from build123d import *

# Parameters (mm, degrees)
SKETCH1_W           = 80
SKETCH1_H           = 24.7
BOSS_EXTRUDE1_DEPTH = 1
CUT_EXTRUDE1_DEPTH  = 100
CUT_EXTRUDE2_DEPTH  = 1
BOSS_EXTRUDE2_START = -80
BOSS_EXTRUDE2_DEPTH = 80


with BuildPart() as part:
    # Sketch1 → Boss-Extrude1 (new body)
    with BuildSketch(Plane.XY):
        Rectangle(SKETCH1_W, SKETCH1_H)
    extrude(amount=BOSS_EXTRUDE1_DEPTH)

    # Sketch2 → Cut-Extrude1 (cut)
    with BuildSketch(Plane.ZY.offset(40)):
        with BuildLine():
            Line((0, -12.35), (1, -12.35))
            ThreePointArc((1, -12.35), (0.292893219, -12.057106781), (0, -11.35))
            Line((0, -11.35), (0, -12.35))
        make_face()
    extrude(amount=-CUT_EXTRUDE1_DEPTH, mode=Mode.SUBTRACT)

    # Sketch3 → Cut-Extrude2 (cut)
    with BuildSketch(Plane(origin=(0, 0, 0), x_dir=(-1, 0, 0), z_dir=(0, 0, -1))):
        with BuildLine():
            Line((34, 7.35), (16, 7.35))
            ThreePointArc((16, 7.35), (15.292893219, 7.057106781), (15, 6.35))
            Line((15, 6.35), (15, -1.65))
            ThreePointArc((15, -1.65), (15.292893219, -2.357106781), (16, -2.65))
            Line((16, -2.65), (34, -2.65))
            ThreePointArc((34, -2.65), (34.707106781, -2.357106781), (35, -1.65))
            Line((35, -1.65), (35, 6.35))
            ThreePointArc((35, 6.35), (34.707106781, 7.057106781), (34, 7.35))
        make_face()
    extrude(amount=-CUT_EXTRUDE2_DEPTH, mode=Mode.SUBTRACT)

    # Sketch4 → Boss-Extrude2 (add)
    with BuildSketch(Plane(origin=(40, 0, 0), x_dir=(0, 0, -1), z_dir=(1, 0, 0)).offset(BOSS_EXTRUDE2_START)):
        with BuildLine():
            Line((-1, -12.49), (-1, -12.35))
            ThreePointArc((-1, -12.35), (-0.292893219, -12.057106781), (0, -11.35))
            Line((0, -11.35), (0.14, -11.35))
            ThreePointArc((0.14, -11.35), (-0.193898269, -12.156101731), (-1, -12.49))
        make_face()
    extrude(amount=BOSS_EXTRUDE2_DEPTH)


solid = part.part
Geometry: final body of the model. Coordinates: model frame, mm. A direction names the side the tool comes from. Give positions to 0.01 mm unless a question says otherwise; leave off trailing zeros. Write each loop counter-clockwise with the first axis right and the second up, starting at its lowest first coordinate (ties: lowest second). Pieces come first, ordered by that corner, then holes.
(1) Cut plane A-A, the plane y = 5.25. Return loops of the section in (x, z), then the cut area to 3 significant figures.
(2) Cut plane D-D, the plane x = -6.5. Return loops of the section in (y, z).
(3) Cut plane B-B, the plane x = -28. Return loops of the section in (y, z), then the cut area to 3 significant figures.
(4) Cut plane C-C, the plane z = 0.4. Return loops of the section in (x, y).
(5) Access query for faces 1 (the flat face through (-1, 0, 1)), 2 (the flat face through (-1, 1, 0)). Directions: +Z, -Z, +X, -X, +Y, -Y. A direction counts if a zero-diameter tool reaches every point of the face in a straight line with its end or side. Return the directions, or none.
(6) Ray query, line 1 (X direction, y = 3, z = 0.4); line 2 (Y direction, x = -3.5, z = 0.9); line 3 (Z direction, x = 23, y = -4.5). Return the intervals inside material, ascending.
Values follow:
1. outline: (-40, 0) - (-35, 0) - (-35, 1) - (-40, 1) - close; (-15, 0) - (40, 0) - (40, 1) - (-15, 1) - close
1. area: 60.0 mm2
2. outline: (-12.49, 1) arc R1.14 ccw to (-11.35, -0.14) - (-11.35, 0) - (12.35, 0) - (12.35, 1) - close
3. outline: (-12.49, 1) arc R1.14 ccw to (-11.35, -0.14) - (-11.35, 0) - (-2.65, 0) - (-2.65, 1) - close; (7.35, 0) - (12.35, 0) - (12.35, 1) - (7.35, 1) - close
3. area: 14.7 mm2
4. outline: (-40, -12.32) - (40, -12.32) - (40, 12.35) - (-40, 12.35) - close; hole (-35, -1.65) arc R1 ccw to (-34, -2.65) - (-16, -2.65) arc R1 ccw to (-15, -1.65) - (-15, 6.35) arc R1 ccw to (-16, 7.35) - (-34, 7.35) arc R1 ccw to (-35, 6.35) - close
5. face 1: +Z, +X, -X, +Y, -Y
5. face 2: -Z, +X, -X, +Y
6. line 1: x = -40 to -35, -15 to 40
6. line 2: y = -12.49 to 12.35
6. line 3: z = 0 to 1
